from build123d import *

# Parameters (mm, degrees)
SKETCH1_W                       = 102
SKETCH1_H                       = 38
BOSS_EXTRUDE1_DEPTH             = 25
SKETCH2_R                       = 3
CUT_EXTRUDE1_DEPTH              = 60
M4X0_7_TAPPED_HOLE1_D           = 3.3
M4X0_7_TAPPED_HOLE1_DEPTH       = 8.1
M4X0_7_TAPPED_HOLE1_CSINK_D     = 4.05
M4X0_7_TAPPED_HOLE1_CSINK_ANGLE = 100
M4X0_7_TAPPED_HOLE1_TIP         = 0.991420021


with BuildPart() as part:
    # Sketch1 → Boss-Extrude1 (new body)
    with BuildSketch(Plane.XY):
        with Locations((51, 19)):
            Rectangle(SKETCH1_W, SKETCH1_H)
    extrude(amount=BOSS_EXTRUDE1_DEPTH)

    # Sketch2 → Cut-Extrude1 (cut)
    with BuildSketch(Plane.ZY):
        with Locations((12.5, 19)):
            Circle(SKETCH2_R)
    extrude(amount=-CUT_EXTRUDE1_DEPTH, mode=Mode.SUBTRACT)

    # M4x0.7 Tapped Hole1
    with Locations(Plane(origin=(0, 0, 0), x_dir=(-1, 0, 0), z_dir=(0, -1, 0))):
        with Locations((-82, -4), (-12, -4), (-12, -21), (-82, -21)):
            CounterSinkHole(M4X0_7_TAPPED_HOLE1_D / 2, M4X0_7_TAPPED_HOLE1_CSINK_D / 2, depth=M4X0_7_TAPPED_HOLE1_DEPTH, counter_sink_angle=M4X0_7_TAPPED_HOLE1_CSINK_ANGLE)
            with Locations((0, 0, -(M4X0_7_TAPPED_HOLE1_DEPTH + M4X0_7_TAPPED_HOLE1_TIP / 2))):  # 118° drill point
                Cone(0, M4X0_7_TAPPED_HOLE1_D / 2, M4X0_7_TAPPED_HOLE1_TIP, mode=Mode.SUBTRACT)


solid = part.part
Can you work these out from the model? Positions are in its coordinate system, mm. A direction names the side the tool comes from. Give positions to 0.01 mm unless a question says otherwise; leave off trailing zeros. Loops run counter-clockwise (first coordinate to the right, second up) from the corner with the lowest first, then second, coordinate; pieces in that order, holes last. Notation, with made-up numbers: (15, -23.75) - (72, -23.75) arc R20 ccw to (72, -19.75) - close; hole circle Ø9 at (8, 43). An arc over 180 degrees is marked (long way). Return JSON: item names as keys, results as strings.
1. I want a section at A-A on x = 27. Please give me the cut outline in (y, z), and give its area (3 significant figures).
Output values:
{"outline": "(0, 0) - (38, 0) - (38, 25) - (0, 25) - close; hole circle Ø6 at (19, 12.5)", "area": "922 mm²"}
2. If I drill on line 1 (X direction, y = 5.5, z = 21); line 2 (Z direction, x = 82, y = 3.5); line 3 (Y direction, x = 40.5, z = 11), over which ranges is the centre line in solid material (lowest first)?
Output values:
{"line 1": "x = 0 to 10.35, 13.65 to 80.35, 83.65 to 102", "line 2": "z = 0 to 2.35, 5.65 to 19.35, 22.65 to 25", "line 3": "y = 0 to 16.4, 21.6 to 38"}
3. We'd pull the mould along X, two halves only. Please class faces 4 (the face through (12.04, 8.92, 20.72)), 5 (the face through (102, 19, 12)), 6 (the face through (60, 19, 12)): +X half, -X half, draft (parallel to the pull), parting line (faces both ways), or undercut.
Output values:
{"face 4": "undercut", "face 5": "+X half", "face 6": "-X half"}
4. I'm going to push flat-ended pins straight in: pin 1 Ø2.5 at (x, z) = (82, 21) entering from -Y; pin 2 Ø5.5 at (y, z) = (19, 12.5) entering from -X. Where does each tip first touch, or does it pass through?
Output values:
{"pin 1": "stops at y = 8.34", "pin 2": "stops at x = 60"}
5. For faces 1 (the face through (0, 15, 12)), 2 (the face through (80.784, 4.262, 19.885)), 3 (the face through (29.6, 17.2, 10.1)), which set-ups out of +Z, -Z, +X, -X, +Y, -Y let a thin tool reach every point of the face, with its end or its side?
Output values:
{"face 1": "+Z, -Z, -X, +Y, -Y", "face 2": "-Y", "face 3": "-X"}
6. I want a section at C-C on z = 12.5. Please give me the cut outline in (x, y).
Output values:
{"outline": "(0, 0) - (102, 0) - (102, 38) - (0, 38) - (0, 22) - (60, 22) - (60, 16) - (0, 16) - close"}
7. I want a section at B-B on y = 19. Please give me the cut outline in (x, z), and give its area (3 significant figures).
Output values:
{"outline": "(0, 0) - (102, 0) - (102, 25) - (0, 25) - (0, 15.5) - (60, 15.5) - (60, 9.5) - (0, 9.5) - close", "area": "2,190 mm²"}
